```python
from build123d import *

# Parameters (mm, degrees)
SKETCH1_R            = 2
BOSS_EXTRUDE1_DEPTH  = 12
SKETCH2_R            = 2.5
BOSS_EXTRUDE2_DEPTH  = 1
FILLET1_R            = 0.5
FILLET1_OF_MIRROR1_R = 0.5


with BuildPart() as part:
    # Sketch1 → Boss-Extrude1 (new body)
    with BuildSketch(Plane(origin=(0, 0, 0), x_dir=(0, 0, -1), z_dir=(1, 0, 0))):
        Circle(SKETCH1_R)
    extrude(amount=BOSS_EXTRUDE1_DEPTH)

    # Sketch2 → Boss-Extrude2 (add)
    with BuildSketch(Plane.ZY):
        Circle(SKETCH2_R)
    boss_extrude2 = extrude(amount=BOSS_EXTRUDE2_DEPTH)

    # Fillet1
    fillet1_edges = [part.edges().sort_by_distance(p)[0] for p in [
        (-1, 0, -2.5),
    ]]
    fillet(fillet1_edges, radius=FILLET1_R)

    # Mirror1: Boss-Extrude2 across plane
    add(boss_extrude2.mirror(Plane(origin=(6, 0, 0), x_dir=(0, 0, 1), z_dir=(1, 0, 0))))

    # Fillet1 of Mirror1
    fillet1_of_mirror1_edges = [part.edges().sort_by_distance(p)[0] for p in [
        (13, 0, -2.5),
    ]]
    fillet(fillet1_of_mirror1_edges, radius=FILLET1_OF_MIRROR1_R)


solid = part.part
```
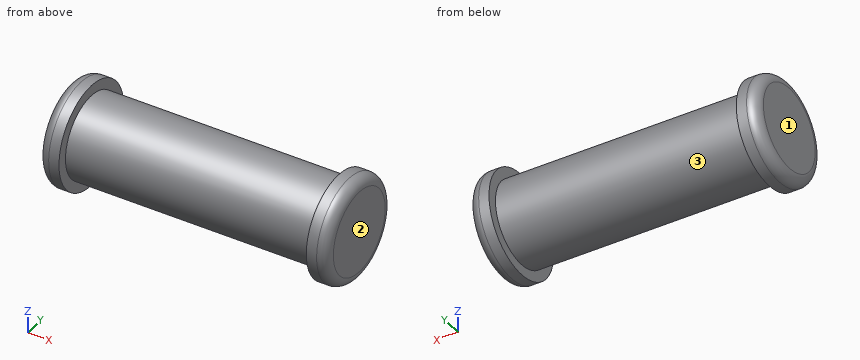
Input: part model. Units: mm. Frame: model coordinates. Face numbers are marked on the shaded views. Give positions to 0.01 mm unless a question says otherwise; leave off trailing zeros. Order: outer loops, then holes, each group sorted by start corner. A loop starts at its lowest first (then second) coordinate and runs counter-clockwise, first axis right, second up. Notation, with made-up numbers: M -25,27.5 L 10,27.5 A16 ccw 10,39.5 Z; hole C -39,-35 d10. An arc over 180 degrees is marked long. Return JSON: item names as keys, results as strings.
1) Section query C-C on x = 7.75. Output: boundary loops of the cut face in (y, z).
Taken from the geometry:
{"outline": "C 0,0 d4"}
2) Section query A-A on y = 0. Output: boundary loops of the cut face in (x, z).
Taken from the geometry:
{"outline": "M -1,-2 A0.5 ccw -0.5,-2.5 L 0,-2.5 L 0,-2 L 12,-2 L 12,-2.5 L 12.5,-2.5 A0.5 ccw 13,-2 L 13,2 A0.5 ccw 12.5,2.5 L 12,2.5 L 12,2 L 0,2 L 0,2.5 L -0.5,2.5 A0.5 ccw -1,2 Z"}
3) Line query: L1, parallel to Y at x = 8.75, z = -0.05; L2, parallel to X at y = 0.95, z = -1.85; L3, parallel to X at y = 2, z = -1. Output: solid intervals per line, ascending. Write a range as [from, to].
Taken from the geometry:
{"L1": "y = [-2, 2]", "L2": "x = [-0.99, 0], [12, 12.99]", "L3": "x = [-0.94, 0], [12, 12.94]"}
4) Mould query, pull axis X, two halves, no side actions, for the marked faces 1, 2 and 3. Classes: released by +X, released by -X, zero draft, split by the parting line, or undercut.
Taken from the geometry:
{"face 1": "released by -X", "face 2": "released by +X", "face 3": "undercut"}
5) Contact query for a flat-ended pin moving along its axis: pin 1 (1.5 mm diameter, centred on x = 2, y = -1.5, fed in from -Z). Output: stop coordinate, or through.
Taken from the geometry:
{"pin 1": "stops at z = -1.85"}
